Source: CAD feature listing. Evaluate the final solid. Frame: model axes, mm. A direction names the side the tool comes from. Give positions to 0.01 mm unless a question says otherwise; leave off trailing zeros. Write each loop counter-clockwise with the first axis right and the second up, starting at its lowest first coordinate (ties: lowest second). Pieces come first, ordered by that corner, then holes. Notation, with made-up numbers: (61, 9) -> (102, 9) arc R19 cw to (102, 24) -> close; hole circle Ø4 at (-31.75, 60.5). An arc over 180 degrees is marked (long way). Use a Markdown table: item, result. Add a question column.
```python
from build123d import *

# Parameters (mm, degrees)
F1_DEPTH = 40


with BuildPart() as f1:
    # F0 (on Front) → F1 (new body)
    with BuildSketch(Plane.XZ):
        with BuildLine():
            Line((6.492765, 26.425125), (-8.507235, 26.425125))
            Line((-8.507235, 26.425125), (-8.507235, -8.574875))
            Line((-8.507235, -8.574875), (-1.007235, -8.574875))
            ThreePointArc((-1.007235, -8.574875), (13.992765, 6.425125), (28.992765, -8.574875))
            Line((28.992765, -8.574875), (36.492765, -8.574875))
            Line((36.492765, -8.574875), (36.492765, 26.425125))
            Line((36.492765, 26.425125), (21.492765, 26.425125))
            Line((21.492765, 26.425125), (21.492765, 16.425125))
            Line((21.492765, 16.425125), (6.492765, 16.425125))
            Line((6.492765, 16.425125), (6.492765, 26.425125))
        make_face()
    extrude(amount=F1_DEPTH)


solid = f1.part
```
(1) Cut plane D-D on x = 12. Return the cut outline in (y, z).
(2) Cut plane B-B on y = -27. Return the cut outline in (x, z).
(3) Material intervals for L1, parallel to X at y = -26, z = 17.5; L2, parallel to X at y = -32.5, z = -4; L3, parallel to Z at x = 0.5, y = -32, sorted ascending.
(4) Cut plane A-A on z = 21.5. Return the cut outline in (x, y).
(5) Access query for faces 1 (the flat face through (21.493, -20, 21)), 2 (the flat face through (-5, -20, -8.575)). Directions: +Z, -Z, +X, -X, +Y, -Y. A direction counts if a zero-diameter tool reaches every point of the face in a straight line with its end or side. Return the directions, or none.
(6) First-contact query: pin 1 Ø1 at (x, y) = (17.5, -34.5) entering from +Z; pin 2 Ø2 at (x, y) = (5.5, -22.5) entering from -Z. Flat tips, straight axial feed; report the tip coordinate or a pass-through.
(7) Mould query, pull axis X, two halves, no side actions, for faces 3 (the cylindrical face through (13.66, -19.72, 6.42)), 4 (the flat face through (14, -40, 9)), 5 (the flat face through (36.493, -20, 9)). Classes: +X half, -X half, draft (parallel to the pull), parting line (faces both ways), or undercut.
(8) Cut plane C-C on z = 4. Return the cut outline in (x, y), then the cut area to 3 significant figures.
Output:
| question | item | result |
|---|---|---|
| 1 | outline | (-40, 6.29) -> (0, 6.29) -> (0, 16.43) -> (-40, 16.43) -> close |
| 2 | outline | (-8.51, -8.57) -> (-1.01, -8.57) arc R15 cw to (28.99, -8.57) -> (36.49, -8.57) -> (36.49, 26.43) -> (21.49, 26.43) -> (21.49, 16.43) -> (6.49, 16.43) -> (6.49, 26.43) -> (-8.51, 26.43) -> close |
| 3 | L1 | -8.51 to 6.49, 21.49 to 36.49 |
| 3 | L2 | -8.51 to -0.29, 28.28 to 36.49 |
| 3 | L3 | -2.02 to 26.43 |
| 4 | outline | (-8.51, -40) -> (6.49, -40) -> (6.49, 0) -> (-8.51, 0) -> close; (21.49, -40) -> (36.49, -40) -> (36.49, 0) -> (21.49, 0) -> close |
| 5 | face 1 | +Z, +Y, -Y |
| 5 | face 2 | -Z, +X, -X, +Y, -Y |
| 6 | pin 1 | z = 16.43 |
| 6 | pin 2 | z = 3.04 |
| 7 | face 3 | undercut |
| 7 | face 4 | draft |
| 7 | face 5 | +X half |
| 8 | outline | (-8.51, -40) -> (5.82, -40) -> (5.82, 0) -> (-8.51, 0) -> close; (22.17, -40) -> (36.49, -40) -> (36.49, 0) -> (22.17, 0) -> close |
| 8 | area | 1,150 mm^2 |
